Autodesk Inventor part; units mm, degrees
ref_plane "YZ Plane" through (0, 0, 0) normal (1, 0, 0) x (0, 1, 0)
ref_plane "XZ Plane" through (0, 0, 0) normal (0, 1, 0) x (-1, 0, 0)
ref_plane "XY Plane" through (0, 0, 0) normal (0, 0, 1) x (1, 0, 0)
sketch "Sketch1" plane through (0, 0, 0) normal (0, 1, 0) x (-1, 0, 0)
  circle A0 centre (0, 0) radius 1.675
  dimension "d0" = 3.35
extrude "Extrusion1" add sketch "Sketch1" along normal blind 20
sketch "Sketch2" plane through (0, 20, 0) normal (0, 1, 0) x (1, 0, 0)
  circle A0 centre (0, 0) radius 1.675
  circle A1 centre (0, 0) radius 2.925
  dimension "d3" = 5.85
extrude "Extrusion2" add sketch "Sketch2" along normal blind 3 contours A0 | A1
sketch "Sketch3" plane through (0, 23, 0) normal (0, 1, 0) x (1, 0, 0)
  line L0 (-0.8268, 1.1831) -> (0.6112, 1.3076)
  line L1 (0.6112, 1.3076) -> (1.438, 0.1244)
  line L2 (1.438, 0.1244) -> (0.8268, -1.1831)
  line L3 (0.8268, -1.1831) -> (-0.6112, -1.3076)
  line L4 (-0.6112, -1.3076) -> (-1.438, -0.1244)
  line L5 (-1.438, -0.1244) -> (-0.8268, 1.1831)
  point P0 (0, 0)
  point P1 (0, 0)
  dimension "d6" = 2.5
extrude "Extrusion3" cut sketch "Sketch3" against normal blind 1.9
equation "\"d0\" = M3_A"
equation "\"d3\" = M3_B"
properties part number "M3_SCREW_20MM"
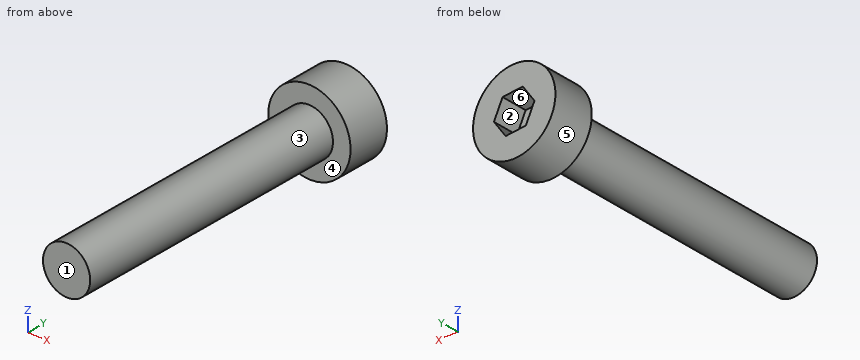
CAD build for the part. Positions are in the model's coordinates, mm. Face numbers are marked on the shaded views. A direction names the side the tool comes from. Coordinates: 2 decimals unless noted, no trailing zeros. Loops run counter-clockwise (first coordinate to the right, second up) from the corner with the lowest first, then second, coordinate; pieces in that order, holes last. Notation, with made-up numbers: (4.25, 66) - (36.25, 66) arc R24 ccw to (36.25, 81) - close; hole circle Ø10 at (50.5, -31.75). An arc over 180 degrees is marked (long way). Use one line per item in the form item = value. Start each with the question number.
1) Band-saw the part on A-A (x = 0). Give the cut face in (y, z) (3 decimals).
2) Two-plate mould, pull along X, no slides. Class the marked faces 4, 5 and 6: +X half, -X half, draft (parallel to the pull), parting line (faces both ways), or undercut.
3) Band-saw the part on B-B (z = 0.65). Give the cut face in (x, y), and give its area (3 significant figures).
4) Flat gauge pins, fed straight in: pin 1 (1.5 mm diameter, centred on y = 19, z = 1.5, fed in from -X); pin 2 (1.5 mm diameter, centred on x = -0.5, y = 2.5, fed in from +Z) (3 decimals); pin 3 (1 mm diameter, centred on y = 11, z = -2.5, fed in from -X); pin 4 (2 mm diameter, centred on x = -1.5, y = 5, fed in from +Z). Where does each tip first touch, or does it go through?
5) Drill centre lines: L1, parallel to Z at x = 0, y = 16.5 (3 decimals); L2, parallel to Y at x = 1.95, z = 0.55; L3, parallel to Y at x = 0.9, z = 0.9. Where is each one in solid material? Low to high. Write a range as from..to.
6) Tool access for the marked faces 1, 2 and 3: list every direction of +Z, -Z, +X, -X, +Y, -Y with a clear straight run to the whole face (end or side of a thin tool).
7) Band-saw the part on C-C (y = 13). Give the cut face in (x, z) (3 decimals), and give its area (3 significant figures).
8) Band-saw the part on D-D (z = 2.3). Give the cut face in (x, y), and give its area (3 significant figures).
Check values:
q1.outline = (0, -1.675) - (20, -1.675) - (20, -2.925) - (23, -2.925) - (23, -1.255) - (21.1, -1.255) - (21.1, 1.255) - (23, 1.255) - (23, 2.925) - (20, 2.925) - (20, 1.675) - (0, 1.675) - close
q2.face_4 = draft
q2.face_5 = parting line
q2.face_6 = undercut
q3.outline = (-2.85, 20) - (-1.54, 20) - (-1.54, 0) - (1.54, 0) - (1.54, 20) - (2.85, 20) - (2.85, 23) - (1.08, 23) - (1.08, 21.1) - (-1.07, 21.1) - (-1.07, 23) - (-2.85, 23) - close
q3.area = 74.8 mm2
q4.pin_1 = -1.5
q4.pin_2 = 1.675
q4.pin_3 = through
q4.pin_4 = 1.6
q5.L1 = -1.675..1.675
q5.L2 = 20..23
q5.L3 = 0..21.1
q6.face_1 = +Z, -Z, +X, -X, -Y
q6.face_2 = +Y
q6.face_3 = -Y
q7.outline = circle Ø3.35 at (0, 0)
q7.area = 8.81 mm2
q8.outline = (-1.81, 20) - (1.81, 20) - (1.81, 23) - (-1.81, 23) - close
q8.area = 10.8 mm2
